Verification items for the finished model (mm, model axes). Face numbers are marked on the shaded views. A direction names the side the tool comes from. Round coordinates to 2 decimals unless told otherwise and drop trailing zeros. Order: outer loops, then holes, each group sorted by start corner. A loop starts at its lowest first (then second) coordinate and runs counter-clockwise, first axis right, second up. Notation, with made-up numbers: M 8,66.25 L 42,66.25 A26 cw 42,105.25 Z; hole C 55,18 d11. An arc over 180 degrees is marked long. One line per item, written item: value. Start each with the question number.
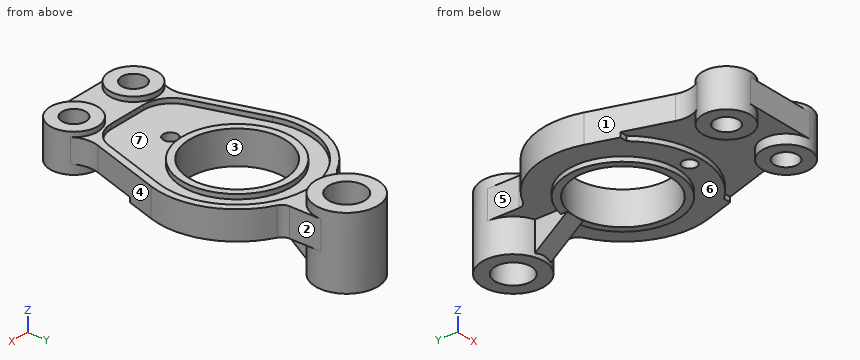
from build123d import *

# Parameters (mm, degrees)
SKETCH1_R               = 50
BOSS_EXTRUDE1_DEPTH     = 35
BOSS_EXTRUDE2_START     = 5
SKETCH1_4_R             = 25
SKETCH1_4_R_2           = 12.5
BOSS_EXTRUDE2_DEPTH     = 40
BOSS_EXTRUDE3_START     = 10
SKETCH1_5_R             = 32.5
BOSS_EXTRUDE3_DEPTH     = 75
SKETCH2_R               = 57.5
CUT_EXTRUDE1_DEPTH      = 5
FILLET1_R               = 10
CUT_EXTRUDE2_START      = -5
CUT_EXTRUDE2_OUTLINE_R  = 57.5
CUT_EXTRUDE2_DEPTH      = 5
CUT_EXTRUDE2_START_2    = -35
CUT_EXTRUDE2_2_DEPTH    = 30
CUT_EXTRUDE3_DEPTH      = 302.76563754
CUT_EXTRUDE3_DEPTH_BACK = 5
RIB1_REACH              = 308.084
SKETCH5_WALL_W          = 655.171326186
SKETCH5_WALL_H          = 20
CUT_EXTRUDE4_DEPTH      = 307.084138759
CUT_EXTRUDE4_DEPTH_BACK = 307.084138759
SKETCH1_6_R             = 12.5
SKETCH1_6_R_2           = 19


# Read off the part's stored shape, not the designer's step: Cut-Extrude2, Ø15.0 (15) Diameter Hole1
with BuildPart() as part:
    # Sketch1 → Boss-Extrude1 (new body)
    with BuildSketch(Plane.XY):
        with BuildLine():
            ThreePointArc((-32.5, 215.828754441), (-74.981933284, 174.408715189), (-78.681648437, 115.191771541))
            Line((-78.681648437, 115.191771541), (-49.309407385, 22.034924488))
            ThreePointArc((-49.309407385, 22.034924488), (-61.74740308, -6.087975353), (-37.5, -25))
            Line((-37.5, -25), (37.5, -25))
            ThreePointArc((37.5, -25), (61.74740308, -6.087975353), (49.309407385, 22.034924488))
            Line((49.309407385, 22.034924488), (78.681648437, 115.191771541))
            ThreePointArc((78.681648437, 115.191771541), (74.981933284, 174.408715189), (32.5, 215.828754441))
            Line((32.5, 215.828754441), (32.5, 255))
            ThreePointArc((32.5, 255), (0, 287.5), (-32.5, 255))
            Line((-32.5, 255), (-32.5, 215.828754441))
        make_face()
        with Locations((0, 140)):
            Circle(SKETCH1_R, mode=Mode.SUBTRACT)
    extrude(amount=-BOSS_EXTRUDE1_DEPTH)

    # Sketch1<4> → Boss-Extrude2 (add)
    # profile 1 of 3: a face of its own
    with BuildSketch(Plane.XY.offset(BOSS_EXTRUDE2_START)):
        with Locations((-37.5, 0)):
            Circle(SKETCH1_4_R)
        with Locations((-37.5, 0)):
            Circle(SKETCH1_4_R_2, mode=Mode.SUBTRACT)
    # profile 2 of 3: a face of its own
    with BuildSketch(Plane.XY.offset(BOSS_EXTRUDE2_START)):
        with Locations((-37.5, 0)):
            Circle(SKETCH1_4_R_2)
    # profile 3 of 3: a face of its own
    with BuildSketch(Plane.XY.offset(BOSS_EXTRUDE2_START)):
        with Locations((37.5, 0)):
            Circle(SKETCH1_4_R)
    extrude(amount=-BOSS_EXTRUDE2_DEPTH)

    # Sketch1<5> → Boss-Extrude3 (add)
    with BuildSketch(Plane.XY.offset(BOSS_EXTRUDE3_START)):
        with Locations((0, 255)):
            Circle(SKETCH1_5_R)
    extrude(amount=-BOSS_EXTRUDE3_DEPTH)

    # Sketch2 → Cut-Extrude1 (cut)
    with BuildSketch(Plane.XY):
        with BuildLine():
            Line((-71.528771306, 117.447065037), (-48.994922099, 45.978826015))
            ThreePointArc((-48.994922099, 45.978826015), (-38.122703028, 30.806661872), (-20.383413577, 25))
            Line((-20.383413577, 25), (20.383413577, 25))
            ThreePointArc((20.383413577, 25), (38.122703028, 30.806661872), (48.994922099, 45.978826015))
            Line((48.994922099, 45.978826015), (71.528771306, 117.447065037))
            ThreePointArc((71.528771306, 117.447065037), (0, 215), (-71.528771306, 117.447065037))
        make_face()
        with Locations((0, 140)):
            Circle(SKETCH2_R, mode=Mode.SUBTRACT)
    extrude(amount=-CUT_EXTRUDE1_DEPTH, mode=Mode.SUBTRACT)

    # Fillet1
    fillet1_edges = [part.edges().sort_by_distance(p)[0] for p in [
        (-32.5, 215.828754441, -17.5),
        (32.5, 215.828754441, -17.5),
    ]]
    fillet(fillet1_edges, radius=FILLET1_R)

    # Cut-Extrude2 outline → Cut-Extrude2 (cut)
    with BuildSketch(Plane(origin=(0, 0, -35), x_dir=(-1, 0, 0), z_dir=(0, 0, -1)).offset(CUT_EXTRUDE2_START)):
        with BuildLine():
            Line((-78.681648437, 115.191771541), (-49.309407385, 22.034924488))
            ThreePointArc((-49.309407385, 22.034924488), (-13.25259692, 6.087975353), (-37.5, -25))
            Line((-37.5, -25), (37.5, -25))
            ThreePointArc((37.5, -25), (13.25259692, 6.087975353), (49.309407385, 22.034924488))
            Line((49.309407385, 22.034924488), (78.681648437, 115.191771541))
            ThreePointArc((78.681648437, 115.191771541), (76.179286423, 171.669643512), (37.905405405, 213.276396207))
            ThreePointArc((37.905405405, 213.276396207), (33.957578038, 216.959631177), (32.5, 222.158383626))
            Line((32.5, 222.158383626), (32.5, 255))
            ThreePointArc((32.5, 255), (0, 222.5), (-32.5, 255))
            Line((-32.5, 255), (-32.5, 222.158383626))
            ThreePointArc((-32.5, 222.158383626), (-33.957578038, 216.959631177), (-37.905405405, 213.276396207))
            ThreePointArc((-37.905405405, 213.276396207), (-76.179286423, 171.669643512), (-78.681648437, 115.191771541))
        make_face()
        with Locations((0, 140)):
            Circle(CUT_EXTRUDE2_OUTLINE_R, mode=Mode.SUBTRACT)
    extrude(amount=CUT_EXTRUDE2_DEPTH, mode=Mode.SUBTRACT)

    # Cut-Extrude2 2 outline → Cut-Extrude2 2 (add)
    with BuildSketch(Plane(origin=(0, 0, -35), x_dir=(-1, 0, 0), z_dir=(0, 0, -1)).offset(CUT_EXTRUDE2_START_2)):
        with BuildLine():
            Line((-49.309407385, 22.034924488), (-54.769381812, 39.351751001))
            ThreePointArc((-54.769381812, 39.351751001), (-53.67166818, 26.163789409), (-58.354950152, 13.786625916))
            ThreePointArc((-58.354950152, 13.786625916), (-54.34484107, 18.472989182), (-49.309407385, 22.034924488))
        make_face()
        with BuildLine():
            Line((54.769381812, 39.351751001), (49.309407385, 22.034924488))
            ThreePointArc((49.309407385, 22.034924488), (54.34484107, 18.472989182), (58.354950152, 13.786625916))
            ThreePointArc((58.354950152, 13.786625916), (53.67166818, 26.163789409), (54.769381812, 39.351751001))
        make_face()
    extrude(amount=CUT_EXTRUDE2_2_DEPTH)

    # Sketch4 → Cut-Extrude3 (cut, two sides: drawn at the far end of the back side and taken through both)
    with BuildSketch(Plane(origin=(0, 0, -30), x_dir=(-1, 0, 0), z_dir=(0, 0, -1)).offset(-CUT_EXTRUDE3_DEPTH_BACK)):
        with BuildLine():
            Line((-61.491869381, 85), (-69.162219436, 85))
            Line((-69.162219436, 85), (-54.769381812, 39.351751001))
            ThreePointArc((-54.769381812, 39.351751001), (-53.67166818, 26.163789409), (-58.354950152, 13.786625916))
            ThreePointArc((-58.354950152, 13.786625916), (-15.481080318, 11.839221936), (-37.5, -25))
            Line((-37.5, -25), (37.5, -25))
            ThreePointArc((37.5, -25), (15.481080318, 11.839221936), (58.354950152, 13.786625916))
            ThreePointArc((58.354950152, 13.786625916), (53.67166818, 26.163789409), (54.769381812, 39.351751001))
            Line((54.769381812, 39.351751001), (69.162219436, 85))
            Line((69.162219436, 85), (61.491869381, 85))
            ThreePointArc((61.491869381, 85), (0, 57.5), (-61.491869381, 85))
        make_face()
    extrude(amount=CUT_EXTRUDE3_DEPTH + CUT_EXTRUDE3_DEPTH_BACK, mode=Mode.SUBTRACT)

    # Sketch5 wall → Rib1 (add, up to next)
    with BuildSketch(Plane(origin=(0, 206.25, -47.5), x_dir=(0, -0.792623989105, 0.60971076085), z_dir=(0, -0.60971076085, -0.792623989105)), mode=Mode.PRIVATE) as rib1_sk1:
        Rectangle(SKETCH5_WALL_W, SKETCH5_WALL_H)
    rib1_tool1 = extrude(rib1_sk1.sketch, amount=-RIB1_REACH, mode=Mode.PRIVATE) - part.part
    add(rib1_tool1.solids().sort_by_distance((0, 206.25, -47.5))[0])

    # Sketch1<6> → Cut-Extrude4 (cut, two sides: drawn at the far end of the back side and taken through both)
    with BuildSketch(Plane.XY.offset(-CUT_EXTRUDE4_DEPTH_BACK)):
        with Locations((-37.5, 0)):
            Circle(SKETCH1_6_R)
        with Locations((37.5, 0)):
            Circle(SKETCH1_6_R)
        with Locations((0, 255)):
            Circle(SKETCH1_6_R_2)
    extrude(amount=CUT_EXTRUDE4_DEPTH + CUT_EXTRUDE4_DEPTH_BACK, mode=Mode.SUBTRACT)

    # Ø15.0 (15) Diameter Hole1 outline → Ø15.0 (15) Diameter Hole1 (revolve, cut)
    with BuildSketch(Plane.XZ.offset(-70)):
        Polygon((0, -30), (7.5, -30), (7.5, -5.025), (7.525, -5), (0, -5), align=None)
    revolve(axis=Axis((0, 70, 0), (0, 0, 1)), mode=Mode.SUBTRACT)


solid = part.part
1. Scan lines: line 1 along X through (y, z) = (0, -14.5); line 2 along Y through (x, z) = (0, -21); line 3 along X through (y, z) = (140, -26). Record each from-to range of solid material in increasing order.
2. Section check C-C (x = -44). Give the number of separate pieces and of enclosed holes in the cut face, and give its area (3 significant figures).
3. Section check A-A (y = 140). Record the cut outline in (x, z), and give its area (3 significant figures).
4. Section check B-B (z = -38). Record the cut outline in (x, y), and give its area (3 significant figures).
5. Depth check by flat-ended pin: pin 1 (15 mm diameter, centred on x = 37.5, y = 0, fed in from -Z); pin 2 (2.5 mm diameter, centred on x = -67, z = -26.5, fed in from -Y); pin 3 (12 mm diameter, centred on x = -34.5, z = 2, fed in from -Y); pin 4 (5 mm diameter, centred on x = -10.5, y = 200.5, fed in from +Z). Enter the tip coordinate at first touch or a pass-through.
6. Tool access check on the marked faces 4, 5, 6 and 7. Record the directions out of +Z, -Z, +X, -X, +Y, -Y that give a thin tool (end or side, any length) a straight path to the whole face; none if there is none.
7. Section check D-D (y = 70). Record the cut outline in (x, z) (3 decimals), and give its area (3 significant figures).
8. Draft check along X on the marked faces 1, 2 and 3. Enter one of: released by +X, released by -X, zero draft, split by the parting line, or undercut.
Geometry check:
1. line 1: x = -62.5 to -50, -25 to 25, 50 to 62.5
1. line 2: y = -25 to 62.5, 77.5 to 90, 190 to 236, 274 to 287.5
1. line 3: x = -82.5 to -50, 50 to 82.5
2. separate pieces: 3
2. enclosed holes: 0
2. area: 4,670 mm²
3. outline: M -82.5,-30 L -57.5,-30 L -57.5,-35 L -50,-35 L -50,0 L -57.5,0 L -57.5,-5 L -75,-5 L -75,0 L -82.5,0 Z; M 50,-35 L 57.5,-35 L 57.5,-30 L 82.5,-30 L 82.5,0 L 75,0 L 75,-5 L 57.5,-5 L 57.5,0 L 50,0 Z
3. area: 1,850 mm²
4. outline: M -10,193.9 L 10,193.9 L 10,224.08 A32.5 ccw long -10,224.08 Z; hole C 0,255 d38
4. area: 2,770 mm²
5. pin 1: passes through
5. pin 2: stops at y = 85
5. pin 3: stops at y = -25
5. pin 4: stops at z = -5
6. face 4: +Z, -Z, +X
6. face 5: +Z, -Z, -X, +Y
6. face 6: -Z
6. face 7: +Z
7. outline: M -64.433,-25 L -43.661,-25 L -43.661,-30 L -7.5,-30 L -7.5,-5.025 L -7.525,-5 L -56.569,-5 L -56.569,0 L -64.433,0 Z; M 7.5,-30 L 43.661,-30 L 43.661,-25 L 64.433,-25 L 64.433,0 L 56.569,0 L 56.569,-5 L 7.525,-5 L 7.5,-5.025 Z
7. area: 2,720 mm²
8. face 1: released by -X
8. face 2: released by +X
8. face 3: undercut
